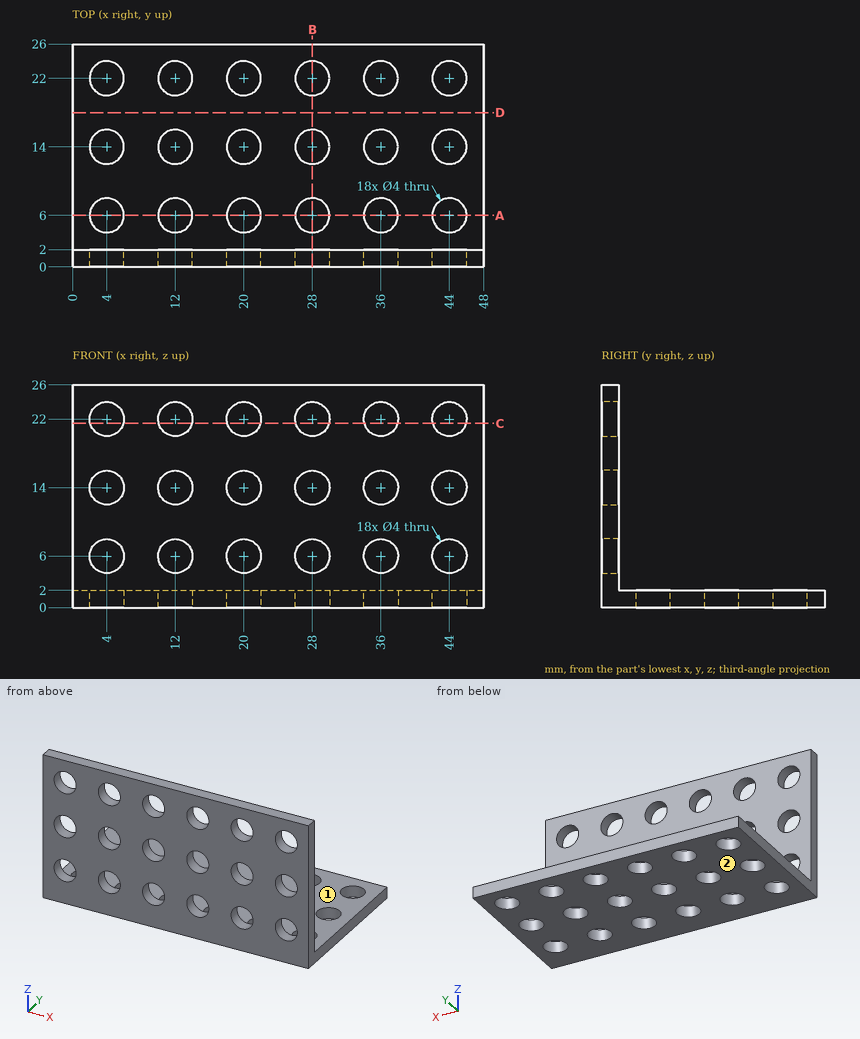
Study the drawing (mm; zero at the part's minimum x, y, z) and answer. A direction names the side the tool comes from. Round coordinates to 2 decimals unless told otherwise and drop trailing zeros. Write each loop counter-clockwise with the first axis right and the second up, starting at its lowest first coordinate (ties: lowest second). Pieces come first, ordered by that corner, then holes. Notation, with made-up numbers: (75, -33.75) - (121, -33.75) arc R25 ccw to (121, -9.75) - close; hole circle Ø11 at (76, -30.75). An arc over 180 degrees is marked (long way). Use a Markdown table: item, result. Add a question column.
1. The part is cut by section D-D (y = 18). Write down the section's boundary in (x, z).
2. Flat-ended cylindrical pins translate along their axes: P1, Ø6.5, axis at x = 44, z = 22, coming from the +Y side; P2, Ø3, axis at x = 12, z = 22, coming from the -Y side; P3, Ø5, axis at x = 28, y = 6, coming from the +Z side; P4, Ø4.5, axis at x = 36, z = 6, coming from the -Y side. Find the tip coordinate at first contact, or state that the pin passes through.
3. The part is cut by section A-A (y = 6). Write down the section's boundary in (x, z), and give its area (3 significant figures).
4. The part is cut by section B-B (x = 28). Give the number of separate pieces and of enclosed holes in the cut face, and give its area (3 significant figures).
5. A tool of negligible diameter and unlimited length cuts with its end or side. For the marked faces 1 and 2, from which of +Z, -Z, +X, -X, +Y, -Y can it reach the whole face along a straight path? Write none if from no direction.
6. Consider line 1 (Y direction, x = 20, z = 0.75); line 2 (Y direction, x = 14.5, z = 17). Determine where each line is inside the solid, lowest interval first.
7. The part is cut by section C-C (z = 21.5). Write down the section's boundary in (x, y).
Reported:
| question | item | result |
|---|---|---|
| 1 | outline | (0, 0) - (48, 0) - (48, 2) - (0, 2) - close |
| 2 | P1 | y = 2 |
| 2 | P2 | through |
| 2 | P3 | z = 2 |
| 2 | P4 | y = 0 |
| 3 | outline | (0, 0) - (2, 0) - (2, 2) - (0, 2) - close; (6, 0) - (10, 0) - (10, 2) - (6, 2) - close; (14, 0) - (18, 0) - (18, 2) - (14, 2) - close; (22, 0) - (26, 0) - (26, 2) - (22, 2) - close; (30, 0) - (34, 0) - (34, 2) - (30, 2) - close; (38, 0) - (42, 0) - (42, 2) - (38, 2) - close; (46, 0) - (48, 0) - (48, 2) - (46, 2) - close |
| 3 | area | 48.0 mm^2 |
| 4 | separate pieces | 7 |
| 4 | enclosed holes | 0 |
| 4 | area | 52.0 mm^2 |
| 5 | face 1 | +Z, +X, -X, +Y |
| 5 | face 2 | -Z, +X, -X, +Y, -Y |
| 6 | line 1 | 0 to 4, 8 to 12, 16 to 20, 24 to 26 |
| 6 | line 2 | 0 to 2 |
| 7 | outline | (0, 0) - (2.06, 0) - (2.06, 2) - (0, 2) - close; (5.94, 0) - (10.06, 0) - (10.06, 2) - (5.94, 2) - close; (13.94, 0) - (18.06, 0) - (18.06, 2) - (13.94, 2) - close; (21.94, 0) - (26.06, 0) - (26.06, 2) - (21.94, 2) - close; (29.94, 0) - (34.06, 0) - (34.06, 2) - (29.94, 2) - close; (37.94, 0) - (42.06, 0) - (42.06, 2) - (37.94, 2) - close; (45.94, 0) - (48, 0) - (48, 2) - (45.94, 2) - close |
